Verification items for the finished model (mm, model axes). A direction names the side the tool comes from. Round coordinates to 2 decimals unless told otherwise and drop trailing zeros. Order: outer loops, then holes, each group sorted by start corner. A loop starts at its lowest first (then second) coordinate and runs counter-clockwise, first axis right, second up. Notation, with made-up numbers: M 81,87.5 L 94,87.5 A22 cw 94,123.5 Z; hole C 29.25,-11 d9. An arc over 180 degrees is marked long. Write item = value, one per line. Start each with the question number.
from build123d import *

# Parameters (mm, degrees)
FILLET1_R                                            = 5
CSK_FOR_M12_HEX_SOCKET_COUNTERSUNK_CAP_S_D           = 13
CSK_FOR_M12_HEX_SOCKET_COUNTERSUNK_CAP_S_CSINK_D     = 26
CSK_FOR_M12_HEX_SOCKET_COUNTERSUNK_CAP_S_CSINK_ANGLE = 90
CSK_FOR_M6_HEX_SOCKET_COUNTERSUNK_CAP_SC_D           = 6.5
CSK_FOR_M6_HEX_SOCKET_COUNTERSUNK_CAP_SC_CSINK_D     = 7.5
CSK_FOR_M6_HEX_SOCKET_COUNTERSUNK_CAP_SC_CSINK_ANGLE = 90
CIRPATTERN1_COUNT                                    = 6


with BuildPart() as part:
    # Sketch1 → Revolve1 (revolve)
    with BuildSketch(Plane.XY, mode=Mode.PRIVATE) as revolve1_sk:
        Polygon((0, 0), (-28, 0), (-28, 35), (-23, 35), (-23, 47.5), (-18, 47.5), (-18, 14), (0, 14), align=None)
    revolve(revolve1_sk.sketch.rotate(Axis((0, 0, 0), (-1, 0, 0)), 90), axis=Axis((0, 0, 0), (-1, 0, 0)))

    # Fillet1
    fillet1_edges = [part.edges().sort_by_distance(p)[0] for p in [
        (-18, 0, 14),
    ]]
    fillet(fillet1_edges, radius=FILLET1_R)

    # CSK for M12 Hex Socket Countersunk Cap Screw1 (through all)
    with Locations(Plane.ZY.offset(28)):
        with Locations((0, 0)):
            CounterSinkHole(CSK_FOR_M12_HEX_SOCKET_COUNTERSUNK_CAP_S_D / 2, CSK_FOR_M12_HEX_SOCKET_COUNTERSUNK_CAP_S_CSINK_D / 2, counter_sink_angle=CSK_FOR_M12_HEX_SOCKET_COUNTERSUNK_CAP_S_CSINK_ANGLE)

    # CSK for M6 Hex Socket Countersunk Cap Screw1 (through all)
    with Locations(Plane(origin=(-18, 0, 0), x_dir=(0, 0, -1), z_dir=(1, 0, 0))):
        with Locations((-40, 0)):
            csk_for_m6_hex_socket_countersunk_cap_sc = CounterSinkHole(CSK_FOR_M6_HEX_SOCKET_COUNTERSUNK_CAP_SC_D / 2, CSK_FOR_M6_HEX_SOCKET_COUNTERSUNK_CAP_SC_CSINK_D / 2, counter_sink_angle=CSK_FOR_M6_HEX_SOCKET_COUNTERSUNK_CAP_SC_CSINK_ANGLE)

    # CirPattern1: CSK for M6 Hex Socket Countersunk Cap Screw1 ×6 about axis
    cirpattern1_axis = Axis((0, 0, 0), (1, 0, 0))
    for i in range(1, CIRPATTERN1_COUNT):
        add(csk_for_m6_hex_socket_countersunk_cap_sc.rotate(cirpattern1_axis, i * 360 / CIRPATTERN1_COUNT), mode=Mode.SUBTRACT)


solid = part.part
1) Scan lines: probe 1 along Y at (x, z) = (-21.7, 20); probe 2 along X at (y, z) = (-35.5, 14.5); probe 3 along X at (y, z) = (32, -5). Record each from-to range of solid material in increasing order.
2) Release check for a two-part mould opening along Z. For faces 1 (the cylindrical face through (-20.782, 1.245, -43.002)), 2 (the flat face through (0, 6, -3)), 3 (the cylindrical face through (-20.78, 37.38, -18.25)), 4 (the cylindrical face through (-20.46, 46.37, 10.3)) record: pulls with the +Z half, pulls with the -Z half, needs draft (parallel to the pull), parting line crosses it, or undercut.
3) Cross-section at B-B, the plane z = 29.5. Enter the section's corners in (x, y).
4) Access from +Z, -Z, +X, -X, +Y, -Y to the whole of each face (thin tool, end or side, straight path). Record for faces 5 (the flat face through (-18, 20, 1)), 6 (the flat face through (-28, 15, 0)).
5) Cross-section at A-A, the plane z = 0. Enter the section's corners in (x, y).
6) Cross-section at C-C, the plane x = -1.75. Enter the section's corners in (y, z).
7) Cross-section at D-D, the plane z = 40. Enter the section's corners in (x, y).
8) Gauge pin test, flat ends, axial feed: P1, Ø1, axis at y = -14, z = 34, coming from the -X side; P2, Ø1.5, axis at x = -23, z = 26.5, coming from the +Y side; P3, Ø8.5, axis at y = 0, z = 40, coming from the +X side. Record the tip position at first contact, or that the pin passes through.
Geometry results:
q1.probe_1 = -43.08 to -37.89, -31.39 to 31.39, 37.89 to 43.08
q1.probe_2 = -23 to -18
q1.probe_3 = -28 to -18
q2.face_1 = undercut
q2.face_2 = needs draft
q2.face_3 = undercut
q2.face_4 = parting line crosses it
q3.outline = M -28,-18.83 L -23,-18.83 L -23,-37.23 L -18,-37.23 L -18,37.23 L -23,37.23 L -23,18.83 L -28,18.83 Z
q4.face_5 = +X
q4.face_6 = +Z, -Z, -X, +Y, -Y
q5.outline = M -28,-35 L -23,-35 L -23,-47.5 L -18,-47.5 L -18,-19 A5 cw -13,-14 L 0,-14 L 0,-6.5 L -21.5,-6.5 L -28,-13 Z; M -28,13 L -21.5,6.5 L 0,6.5 L 0,14 L -13,14 A5 cw -18,19 L -18,47.5 L -23,47.5 L -23,35 L -28,35 Z
q6.outline = C 0,0 d28; hole C 0,0 d13
q7.outline = M -23,-25.62 L -18,-25.62 L -18,-3.75 L -18.5,-3.25 L -23,-3.25 Z; M -23,3.25 L -18.5,3.25 L -18,3.75 L -18,25.62 L -23,25.62 Z
q8.P1 = -23
q8.P2 = 39.91
q8.P3 = -18
